Can you work these out from the model? Positions are in its coordinate system, mm. A direction names the side the tool comes from. Give positions to 0.01 mm unless a question says otherwise; leave off trailing zeros. Order: outer loops, then holes, each group sorted by start corner. A loop starts at its lowest first (then second) coordinate and runs counter-clockwise, first axis right, second up. Notation, with made-up numbers: (48, -32.5) - (87, -32.5) arc R30 ccw to (87, 0.5) - close; hole circle Ø7 at (-4, 4). An arc over 180 degrees is marked (long way). Answer as CSV lines item,"result".
```python
from build123d import *

# Parameters (mm, degrees)
F1_DEPTH = 71.374
F2_R     = 5.08
F3_R     = 6.35
F4_DEPTH = 25.4
F5_DEPTH = 25.4
F6_R     = 3.81
F7_DEPTH = 25.4


with BuildPart() as f1:
    # F0 (on Top) → F1 (new body)
    with BuildSketch(Plane.XY):
        with BuildLine():
            Line((98.164037795, 0), (0, 0))
            Line((0, 0), (-28.835962205, 0))
            Line((-28.835962205, 0), (34.664037795, 63.5))
            Line((34.664037795, 63.5), (31.251540469, 66.912497326))
            Line((31.251540469, 66.912497326), (-35.660956857, 0))
            ThreePointArc((-35.660956857, 0), (-33.661962205, -4.826), (-28.835962205, -6.824994652))
            Line((-28.835962205, -6.824994652), (98.164037795, -6.824994652))
            Line((98.164037795, -6.824994652), (98.164037795, 0))
        make_face()
    extrude(amount=-F1_DEPTH)

    # F2
    f2_edges = [f1.edges().sort_by_distance(p)[0] for p in [
        (32.957789, 65.206249, 0),
        (32.957789, 65.206249, -71.374),
        (98.164038, -3.412497, 0),
        (98.164038, -3.412497, -71.374),
    ]]
    fillet(f2_edges, radius=F2_R)

    # F3 (on face) → F4 (cut)
    with BuildSketch(Plane(origin=(0, 0, 0), x_dir=(-1, 0, 0), z_dir=(0, 1, 0))):
        with Locations((-16.884037795, -35.687)):
            Circle(F3_R)
    extrude(amount=-F4_DEPTH, mode=Mode.SUBTRACT)

    # F3 (on face) → F5 (cut)
    with BuildSketch(Plane(origin=(0, 0, 0), x_dir=(-1, 0, 0), z_dir=(0, 1, 0))):
        with Locations((-16.884037795, -35.687)):
            Circle(F3_R)
        with BuildLine():
            ThreePointArc((-54.984037795, -42.037), (-48.634037795, -35.687), (-54.984037795, -29.337))
            Line((-54.984037795, -29.337), (-80.384037795, -29.337))
            ThreePointArc((-80.384037795, -29.337), (-86.734037795, -35.687), (-80.384037795, -42.037))
            Line((-80.384037795, -42.037), (-54.984037795, -42.037))
        make_face()
    extrude(amount=-F5_DEPTH, mode=Mode.SUBTRACT)

    # F6 (on face) → F7 (cut)
    with BuildSketch(Plane(origin=(-17.8304784285, 17.8304784285, 0), x_dir=(-0.7071067812, -0.7071067812, 0), z_dir=(-0.7071067812, 0.7071067812, 0))):
        with Locations((-50.3624567935, -53.9462038157)):
            Circle(F6_R)
        with Locations((-50.3624567935, -18.4293880287)):
            Circle(F6_R)
    extrude(amount=-F7_DEPTH, mode=Mode.SUBTRACT)


solid = f1.part
```
1) I want a section at A-A on x = 57. Write out the boundary of the cut face in (y, z) (3 decimals).
Answer block:
outline,"(-6.825, -71.374) - (0, -71.374) - (0, -42.037) - (-6.825, -42.037) - close; (-6.825, -29.337) - (0, -29.337) - (0, 0) - (-6.825, 0) - close"
2) I want a section at B-B on z = -17. Write out the boundary of the cut face in (x, y) (1 decimal), plus the area to 3 significant figures.
Answer block:
outline,"(-35.7, 0) arc R6.8 ccw to (-28.8, -6.8) - (98.2, -6.8) - (98.2, 0) - (-28.8, 0) - (18.7, 47.5) - (15.3, 50.9) - close; (20.3, 55.9) - (23.7, 52.5) - (34.7, 63.5) - (31.3, 66.9) - close"
area,"1,310 mm2"
3) If we mould it in two halves opening along Z, with no side actions, what happens to faces 1 (the cylindrical face through (96.72, -3.36, -1.53)), 2 (the cylindrical face through (10.827, -3.365, -33.78)), 3 (the cylindrical face through (31.91, 64.206, -69.846))? For each: +Z half, -Z half, draft (parallel to the pull), parting line (faces both ways), or undercut.
Answer block:
face 1,"+Z half"
face 2,"undercut"
face 3,"-Z half"
4) I want a section at C-C on z = -38. Write out the boundary of the cut face in (x, y) (1 decimal), plus the area to 3 significant figures.
Answer block:
outline,"(-35.7, 0) arc R6.8 ccw to (-28.8, -6.8) - (11, -6.8) - (11, 0) - (-28.8, 0) - (34.7, 63.5) - (31.3, 66.9) - close; (22.8, -6.8) - (49.1, -6.8) - (49.1, 0) - (22.8, 0) - close; (86.3, -6.8) - (98.2, -6.8) - (98.2, 0) - (86.3, 0) - close"
area,"1,010 mm2"
5) I want a section at D-D on z = -59.5. Write out the boundary of the cut face in (x, y) (1 decimal).
Answer block:
outline,"(-35.7, 0) arc R6.8 ccw to (-28.8, -6.8) - (98.2, -6.8) - (98.2, 0) - (-28.8, 0) - (34.7, 63.5) - (31.3, 66.9) - close"
6) Which directions (+Z, -Z, +X, -X, +Y, -Y) give clear straight access to the entire face, cutting with the end or side of a thin tool? Please do faces 4 (the cylindrical face through (48.636, -3.365, -35.827)), 5 (the flat face through (32.982, 65.182, -35.259)), 6 (the flat face through (2.47, 31.306, -35.187)).
Answer block:
face 4,"+Y, -Y"
face 5,"+Z, -Z, +X, +Y"
face 6,"+Z, -Z, +X"
7) I'm going to push flat-ended pins straight in: P1, Ø2, axis at x = -1.5, z = -21, coming from the +Y side; P2, Ø4, axis at y = 4, z = -17.5, coming from the -X side; P3, Ø4, axis at y = 50.5, z = -10, coming from the -X side. Where does each tip first touch, or does it pass through?
Answer block:
P1,"y = 35.16"
P2,"x = -33.66"
P3,"x = 12.84"
8) I need wall thicknesses on line 1 along Y through (x, z) = (37, -41) (3 decimals); line 2 along Y through (x, z) = (-27, -50) (3 decimals); line 3 along Y through (x, z) = (-6, -49) (3 decimals). Which ranges of each line are inside material? Lowest first, please. Write a range as [from, to].
Answer block:
line 1,"[-6.825, 0]"
line 2,"[-6.825, 0], [1.836, 8.661]"
line 3,"[-6.825, 0], [22.836, 29.661]"
